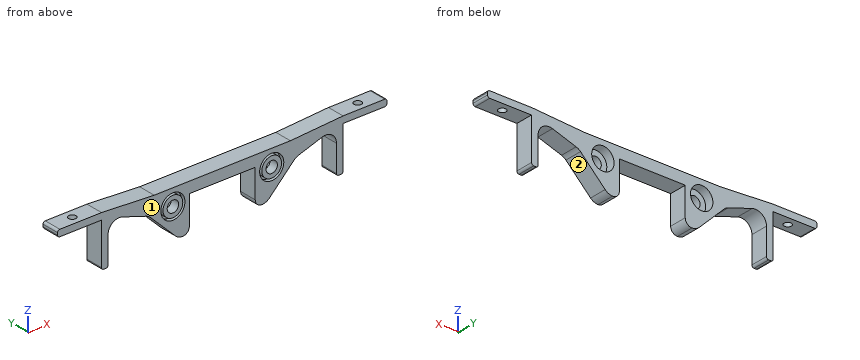
```python
from build123d import *

# Parameters (mm, degrees)
ESQUISSE1_R             = 2.6
BOSS_EXTRU_1_DEPTH      = 8
ESQUISSE3_R             = 5.1
ENL_V_MAT_EXTRU_2_DEPTH = 4
ESQUISSE4_R             = 5.5
ESQUISSE4_R_2           = 4.5
ENL_V_MAT_EXTRU_3_DEPTH = 2
CONG_1_R                = 5
CONG_2_R                = 3
CONG_3_R                = 4
BOSS_EXTRU_2_DEPTH      = 8
CONG_4_R                = 5
ENL_V_MAT_EXTRU_4_REACH = 25
ESQUISSE6_R             = 1.7
CONG_5_R                = 1


with BuildPart() as part:
    # Esquisse1 → Boss.-Extru.1 (new body)
    with BuildSketch(Plane(origin=(0, 0, 0), x_dir=(1, 0, 0), z_dir=(0, 1, 0))):
        Polygon((-35, 0), (35, 0), (35, 6), (20, 21), (15, 21), (15, 5), (-15, 5), (-15, 21), (-20, 21), (-35, 6), align=None)
        with Locations((22.5, 7.5)):
            Circle(ESQUISSE1_R, mode=Mode.SUBTRACT)
        with Locations((-22.5, 7.5)):
            Circle(ESQUISSE1_R, mode=Mode.SUBTRACT)
    extrude(amount=BOSS_EXTRU_1_DEPTH)

    # Esquisse3 → Enlèv. mat.-Extru.2 (cut)
    with BuildSketch(Plane(origin=(0, 8, 0), x_dir=(1, 0, 0), z_dir=(0, 1, 0))):
        with Locations((-22.5, 7.5)):
            Circle(ESQUISSE3_R)
        with Locations((22.5, 7.5)):
            Circle(ESQUISSE3_R)
    extrude(amount=-ENL_V_MAT_EXTRU_2_DEPTH, mode=Mode.SUBTRACT)

    # Esquisse4 → Enlèv. mat.-Extru.3 (cut)
    with BuildSketch(Plane.XZ):
        with Locations((-22.5, -7.5)):
            Circle(ESQUISSE4_R)
        with Locations((-22.5, -7.5)):
            Circle(ESQUISSE4_R_2, mode=Mode.SUBTRACT)
        with Locations((22.5, -7.5)):
            Circle(ESQUISSE4_R)
        with Locations((22.5, -7.5)):
            Circle(ESQUISSE4_R_2, mode=Mode.SUBTRACT)
    extrude(amount=-ENL_V_MAT_EXTRU_3_DEPTH, mode=Mode.SUBTRACT)

    # Congé1
    cong_1_edges = [part.edges().sort_by_distance(p)[0] for p in [
        (-35, 4, -6),
        (-20, 4, -21),
        (20, 4, -21),
        (35, 4, -6),
    ]]
    fillet(cong_1_edges, radius=CONG_1_R)

    # Congé2
    cong_2_edges = [part.edges().sort_by_distance(p)[0] for p in [
        (-15, 4, -21),
        (15, 4, -21),
    ]]
    fillet(cong_2_edges, radius=CONG_2_R)

    # Congé3
    cong_3_edges = [part.edges().sort_by_distance(p)[0] for p in [
        (-35, 4, 0),
        (35, 4, 0),
    ]]
    fillet(cong_3_edges, radius=CONG_3_R)

    # Esquisse5 → Boss.-Extru.2 (add)
    with BuildSketch(Plane(origin=(0, 8, 0), x_dir=(1, 0, 0), z_dir=(0, 1, 0))):
        Polygon((30.997471486, 0), (54.997471486, -1.5), (74.997471486, -1.5), (74.997471486, 1.5), (54.997471486, 1.5), (54.997471486, 21.5), (51.997471486, 21.5), (51.997471486, 1.5), (33.535533906, 7.464466094), align=None)
        Polygon((-33.535533906, 7.464466094), (-30.997471486, 0), (-54.997471486, -1.5), (-74.997471486, -1.5), (-74.997471486, 1.5), (-54.997471486, 1.5), (-54.997471486, 21.5), (-51.997471486, 21.5), (-51.997471486, 1.5), align=None)
    extrude(amount=-BOSS_EXTRU_2_DEPTH)

    # Congé4
    cong_4_edges = [part.edges().sort_by_distance(p)[0] for p in [
        (51.997471486, 4, -1.5),
        (-51.997471486, 4, -1.5),
        (-33.535533906, 4, -7.464466094),
        (33.535533906, 4, -7.464466094),
    ]]
    fillet(cong_4_edges, radius=CONG_4_R)

    # Esquisse6 → Enlèv. mat.-Extru.4 (cut, up to next)
    with BuildSketch(Plane.XY.offset(1.5), mode=Mode.PRIVATE) as enl_v_mat_extru_4_sk1:
        with Locations((64.997471486, 4)):
            Circle(ESQUISSE6_R)
    enl_v_mat_extru_4_tool1 = extrude(enl_v_mat_extru_4_sk1.sketch, amount=-ENL_V_MAT_EXTRU_4_REACH, mode=Mode.PRIVATE) & part.part
    add(enl_v_mat_extru_4_tool1.solids().sort_by_distance((64.997471, 4, 1.5))[0], mode=Mode.SUBTRACT)
    # Esquisse6 → Enlèv. mat.-Extru.4 (cut, up to next)
    with BuildSketch(Plane.XY.offset(1.5), mode=Mode.PRIVATE) as enl_v_mat_extru_4_sk2:
        with Locations((-64.997471486, 4)):
            Circle(ESQUISSE6_R)
    enl_v_mat_extru_4_tool2 = extrude(enl_v_mat_extru_4_sk2.sketch, amount=-ENL_V_MAT_EXTRU_4_REACH, mode=Mode.PRIVATE) & part.part
    add(enl_v_mat_extru_4_tool2.solids().sort_by_distance((-64.997471, 4, 1.5))[0], mode=Mode.SUBTRACT)

    # Congé5
    cong_5_edges = [part.edges().sort_by_distance(p)[0] for p in [
        (51.997471486, 4, -21.5),
        (54.997471486, 4, -21.5),
        (74.997471486, 4, -1.5),
        (74.997471486, 4, 1.5),
        (-74.997471486, 4, 1.5),
        (-74.997471486, 4, -1.5),
        (-54.997471486, 4, -21.5),
        (-51.997471486, 4, -21.5),
    ]]
    fillet(cong_5_edges, radius=CONG_5_R)


solid = part.part
```
Part model, mm, in its own coordinate system. Face numbers are marked on the shaded views. Round coordinates to 2 decimals unless told otherwise and drop trailing zeros. Write each loop counter-clockwise with the first axis right and the second up, starting at its lowest first coordinate (ties: lowest second). Pieces come first, ordered by that corner, then holes.
Item 1: Drop flat-ended pins along their axis: pin 1 Ø9 at (x, z) = (-23, -6.5) entering from -Y; pin 2 Ø4.5 at (x, z) = (22.5, -7.5) entering from +Y; pin 3 Ø1.5 at (y, z) = (2.5, -6.5) entering from +X; pin 4 Ø3 at (y, z) = (4, -6) entering from -X. Give the stop position or say it passes through.
Results:
pin 1: stops at y = 0
pin 2: passes through
pin 3: stops at x = 55
pin 4: stops at x = -55
Item 2: Probe L1, parallel to X at y = 2, z = -13; L2, parallel to Z at x = -22.5, y = 0.5; L3, parallel to X at y = 5.75, z = -19. List the from-to ranges inside material, lowest first.
Results:
L1: x = -55 to -52, -28 to -15, 15 to 28, 52 to 55
L2: z = -18.5 to -13, -12 to -10.1, -4.9 to -3, -2 to 0
L3: x = -55 to -52, -22 to -15.17, 15.17 to 22, 52 to 55
Item 3: Cut at A-A, the plane z = -14.25. Give the cut face in (x, y), plus the area to 3 significant figures.
Results:
outline: (-55, 0) - (-52, 0) - (-52, 8) - (-55, 8) - close; (-26.75, 0) - (-15, 0) - (-15, 8) - (-26.75, 8) - close; (15, 0) - (26.75, 0) - (26.75, 8) - (15, 8) - close; (52, 0) - (55, 0) - (55, 8) - (52, 8) - close
area: 236 mm2
Item 4: Cut at C-C, the plane x = -48. Give the cut face in (y, z).
Results:
outline: (0, -3.47) - (8, -3.47) - (8, 1.06) - (0, 1.06) - close
Item 5: Two-plate mould, pull along X, no slides. Class the marked faces 1 and 2: +X half, -X half, draft (parallel to the pull), parting line (faces both ways), or undercut.
Results:
face 1: draft
face 2: undercut
Item 6: Cut at B-B, the plane x = -7. Give the cut face in (y, z), plus the area to 3 significant figures.
Results:
outline: (0, -5) - (8, -5) - (8, 0) - (0, 0) - close
area: 40.0 mm2
